Geometry check sheet. Reference: drawing and pictorial views, mm from the part's lowest x, y, z. A direction names the side the tool comes from. Coordinates: 2 decimals unless noted, no trailing zeros. Write each loop counter-clockwise with the first axis right and the second up, starting at its lowest first coordinate (ties: lowest second). Pieces come first, ordered by that corner, then holes. Notation, with made-up numbers: (63, 51) - (69, 51) arc R14 ccw to (69, 56) - close; hole circle Ø8 at (65, 80). An arc over 180 degrees is marked (long way). Answer as a JSON object with one key per item and string values. Group by question number.
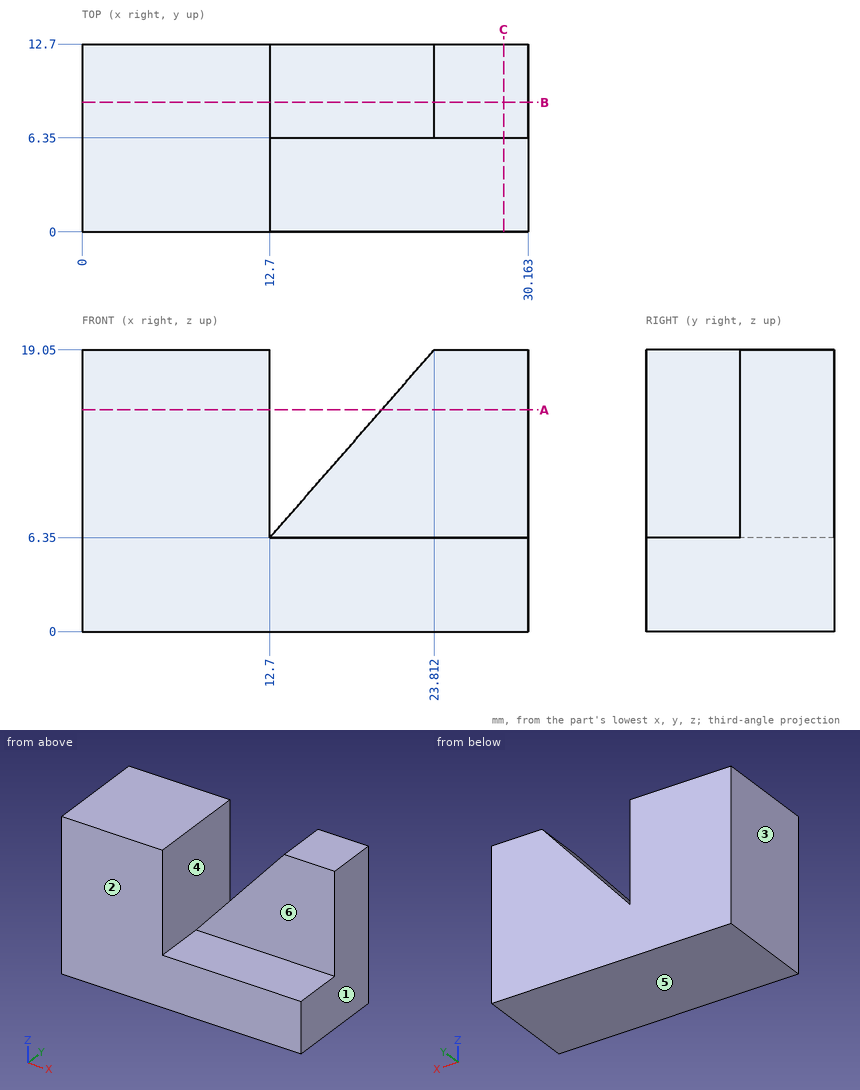
(1) Section check B-B (y = 8.75). Record the cut outline in (x, z).
(2) Material ranges on L1, parallel to Y at x = 15.5, z = 8.75; L2, parallel to X at y = 3.75, z = 12.5; L3, parallel to X at y = 7.75, z = 7.5 (1 decimal), recorded low to high. Write a range as [from, to].
(3) Gauge pin test, flat ends, axial feed: pin 1 (5 mm diameter, centred on x = 19.5, y = 4.5, fed in from +Z) (1 decimal); pin 2 (3 mm diameter, centred on x = 21.5, y = 9, fed in from +Z). Record the tip position at first contact, or that the pin passes through.
(4) Draft check along X on the marked faces 1, 2, 3 and 4. Enter one of: +X half, -X half, draft (parallel to the pull), parting line (faces both ways), or undercut.
(5) Set-up check for the marked faces 5 and 6: record each of +Z, -Z, +X, -X, +Y, -Y from which the full face is reachable in a straight line by a thin tool's end or side.
(6) Section check C-C (x = 28.5). Record the cut outline in (y, z).
(7) Section check A-A (z = 15). Record the cut outline in (x, y).
Conclusion:
{
 "1": {"outline": "(0, 0) - (30.16, 0) - (30.16, 19.05) - (23.81, 19.05) - (12.7, 6.35) - (12.7, 19.05) - (0, 19.05) - close"},
 "2": {"L1": "y = [6.35, 12.7]", "L2": "x = [0, 12.7]", "L3": "x = [0, 12.7], [13.7, 30.2]"},
 "3": {"pin 1": "stops at z = 16", "pin 2": "stops at z = 18.12"},
 "4": {"face 1": "+X half", "face 2": "draft", "face 3": "-X half", "face 4": "undercut"},
 "5": {"face 5": "-Z, +X, -X, +Y, -Y", "face 6": "+Z, +X, -Y"},
 "6": {"outline": "(0, 0) - (12.7, 0) - (12.7, 19.05) - (6.35, 19.05) - (6.35, 6.35) - (0, 6.35) - close"},
 "7": {"outline": "(0, 0) - (12.7, 0) - (12.7, 12.7) - (0, 12.7) - close; (20.27, 6.35) - (30.16, 6.35) - (30.16, 12.7) - (20.27, 12.7) - close"}
}
